Source: three-view drawing plus pictorial views. Frame: mm from the lowest corner of the part. A direction names the side the tool comes from. Round coordinates to 2 decimals unless told otherwise and drop trailing zeros. Order: outer loops, then holes, each group sorted by start corner. A loop starts at its lowest first (then second) coordinate and runs counter-clockwise, first axis right, second up. Notation, with made-up numbers: (36.25, 7) - (73.25, 7) arc R18 cw to (73.25, 36) - close; hole circle Ø8 at (-21, 19.25). An arc over 180 degrees is marked (long way). Use one line per item in the form item = value. Start each with the question number.
Q1. Ray query, line 1 (X direction, y = 201.5, z = 77); line 2 (Z direction, x = 326, y = 478). Return the intervals inside material, ascending. Write a range as [from, to].
Q2. Set-up query: the marked faces 4 and 5. Return all of +Z, -Z, +X, -X, +Y, -Y with unobstructed straight access to the full face (end or side cutting, diameter ignored); none if empty.
Q3. Cut plane B-B, the plane x = 151.5. Return the cut outline in (y, z), and give its area (3 significant figures).
Q4. Cut plane A-A, the plane z = 72. Return the cut outline in (x, y).
Q5. Draft query along X for the marked faces 1, 2 and 3. Return one class per face: released by +X, released by -X, zero draft, split by the parting line, or undercut.
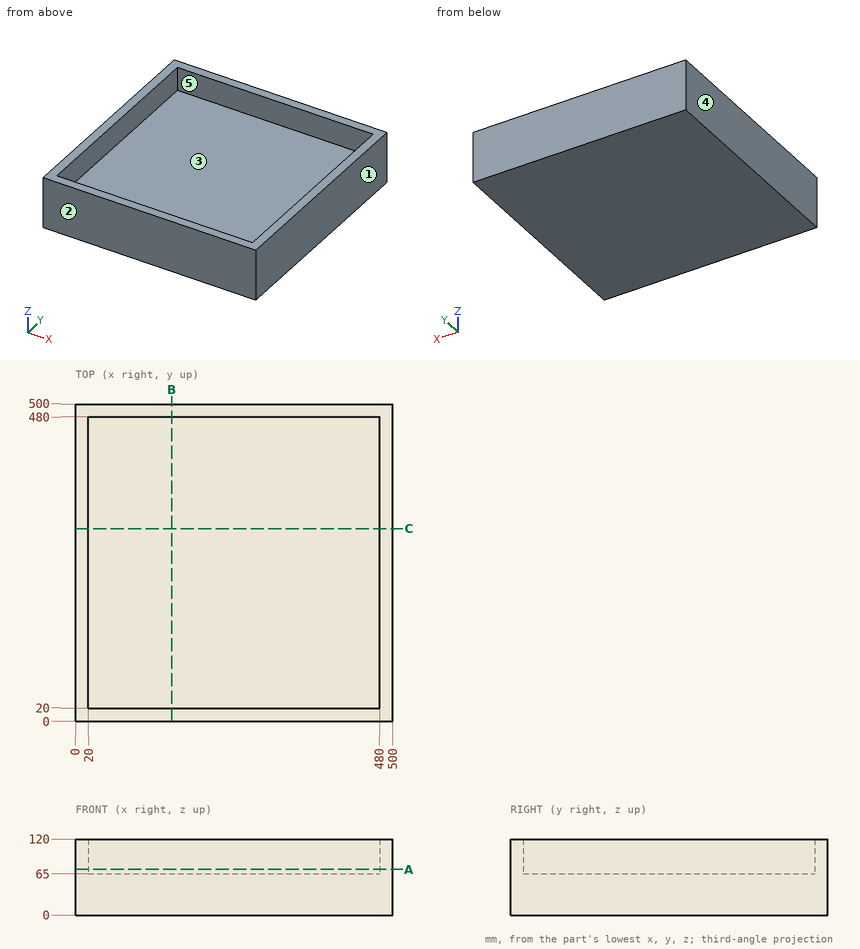
Completed:
q1.line_1 = [0, 20], [480, 500]
q1.line_2 = [0, 65]
q2.face_4 = +Z, -Z, -X, +Y, -Y
q2.face_5 = +Z
q3.outline = (0, 0) - (500, 0) - (500, 120) - (480, 120) - (480, 65) - (20, 65) - (20, 120) - (0, 120) - close
q3.area = 34,700 mm2
q4.outline = (0, 0) - (500, 0) - (500, 500) - (0, 500) - close; hole (20, 20) - (480, 20) - (480, 480) - (20, 480) - close
q5.face_1 = released by +X
q5.face_2 = zero draft
q5.face_3 = undercut
